from build123d import *

# Parameters (mm, degrees)
F0_R      = 18.4
F1_DEPTH  = 24
F2_R      = 17.25
F3_DEPTH  = 30
F4_R      = 6
F5_DEPTH  = 6.5
F6_R      = 3
F7_DEPTH  = 15.5
F8_SIZE   = 1
F10_DEPTH = 12
F12_D     = 3
F12_DEPTH = 24
F12_TIP   = 0.9012909285
F14_DEPTH = 1
F15_R     = 6.5
F16_DEPTH = 1.5
F17_SIZE  = 1
F18_W     = 3.175
F18_H     = 0.79375
F19_DEPTH = 5.6
F20_SIZE  = 1
F22_DEPTH = 25.4
F23_R     = 0.5


with BuildPart() as f1:
    # F0 (on Front) → F1 (new body)
    with BuildSketch(Plane.XZ):
        Circle(F0_R)
    extrude(amount=F1_DEPTH)

    # F2 (on face) → F3 (join)
    with BuildSketch(Plane(origin=(0, 0, 0), x_dir=(-1, 0, 0), z_dir=(0, 1, 0))):
        Circle(F2_R)
    extrude(amount=F3_DEPTH)

    # F4 (on face) → F5 (join)
    with BuildSketch(Plane.XZ.offset(24)):
        with Locations((7, 0)):
            Circle(F4_R)
    extrude(amount=F5_DEPTH)

    # F6 (on face) → F7 (join)
    with BuildSketch(Plane.XZ.offset(30.5)):
        with Locations((7, 0)):
            Circle(F6_R)
    extrude(amount=F7_DEPTH)

    # F8
    f8_edges = [f1.edges().sort_by_distance(p)[0] for p in [
        (1, -30.5, 0),
    ]]
    chamfer(f8_edges, length=F8_SIZE)

    # F9 (on face) → F10 (cut)
    with BuildSketch(Plane.XZ.offset(46)):
        with BuildLine():
            ThreePointArc((8.8, 2.4), (7, 3), (5.2, 2.4))
            Line((5.2, 2.4), (8.8, 2.4))
        make_face()
    extrude(amount=-F10_DEPTH, mode=Mode.SUBTRACT)

    # F12
    with Locations(Plane.XZ.offset(24)):
        with Locations((0, 15.5), (-13.4233937587, 7.75), (-13.4233937587, -7.75), (0, -15.5), (13.4233937587, -7.75), (13.4233937587, 7.75)):
            Hole(F12_D / 2, depth=F12_DEPTH)
            with Locations((0, 0, -(F12_DEPTH + F12_TIP / 2))):  # 118° drill point
                Cone(0, F12_D / 2, F12_TIP, mode=Mode.SUBTRACT)

    # F13 (on face) → F14 (cut)
    with BuildSketch(Plane.XZ.offset(24)):
        with BuildLine():
            ThreePointArc((7.1428571429, 7.9987243881), (8.1017881451, 8.6603638261), (7.7833850932, 9.7810488441))
            ThreePointArc((7.7833850932, 9.7810488441), (-12.5, 0), (7.7833850932, -9.7810488441))
            ThreePointArc((7.7833850932, -9.7810488441), (8.1017881451, -8.6603638261), (7.1428571429, -7.9987243881))
            ThreePointArc((7.1428571429, -7.9987243881), (-1, 0), (7.1428571429, 7.9987243881))
        make_face()
    extrude(amount=-F14_DEPTH, mode=Mode.SUBTRACT)

    # F15 (on face) → F16 (join)
    with BuildSketch(Plane(origin=(0, 30, 0), x_dir=(-1, 0, 0), z_dir=(0, 1, 0))):
        Circle(F15_R)
    extrude(amount=F16_DEPTH)

    # F17
    f17_edges = [f1.edges().sort_by_distance(p)[0] for p in [
        (6.5, 31.5, 0),
    ]]
    chamfer(f17_edges, length=F17_SIZE)

    # F18 (on face) → F19 (join)
    with BuildSketch(Plane(origin=(0, 30, 0), x_dir=(-1, 0, 0), z_dir=(0, 1, 0))):
        with Locations((0, 11.653125)):
            Rectangle(F18_W, F18_H)
        with Locations((0, -11.653125)):
            Rectangle(F18_W, F18_H)
    extrude(amount=F19_DEPTH)

    # F20
    f20_edges = [f1.edges().sort_by_distance(p)[0] for p in [
        (-1.5875, 35.6, 11.653125),
        (1.5875, 35.6, 11.653125),
        (1.5875, 35.6, -11.653125),
        (-1.5875, 35.6, -11.653125),
    ]]
    chamfer(f20_edges, length=F20_SIZE)

    # F21 (on face) → F22 (cut)
    with BuildSketch(Plane.XY.offset(12.05)):
        with BuildLine():
            Line((0.5, 33.04), (0.5, 34.31))
            ThreePointArc((0.5, 34.31), (0, 34.81), (-0.5, 34.31))
            Line((-0.5, 34.31), (-0.5, 33.04))
            ThreePointArc((-0.5, 33.04), (0, 32.54), (0.5, 33.04))
        make_face()
    extrude(amount=-F22_DEPTH, mode=Mode.SUBTRACT)

    # F23
    f23_edges = [f1.edges().sort_by_distance(p)[0] for p in [
        (-18.4, -24, 0),
    ]]
    fillet(f23_edges, radius=F23_R)


solid = f1.part
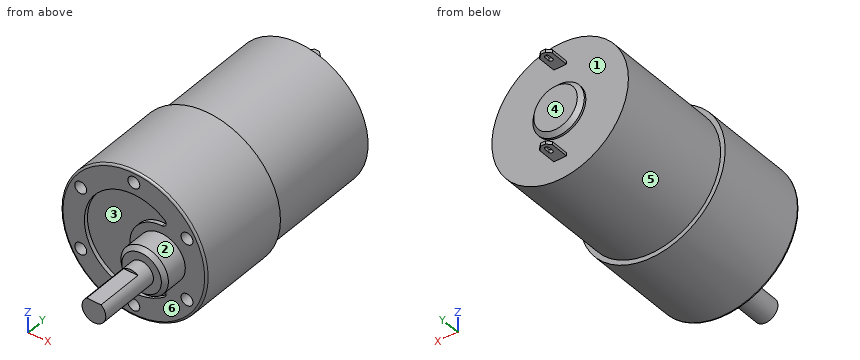
Input: part model. Units: mm. Frame: model coordinates. Face numbers are marked on the shaded views. A direction names the side the tool comes from. Round coordinates to 2 decimals unless told otherwise and drop trailing zeros. Order: outer loops, then holes, each group sorted by start corner. A loop starts at its lowest first (then second) coordinate and runs counter-clockwise, first axis right, second up. Notation, with made-up numbers: (76.25, 5.25) - (125.25, 5.25) arc R5 cw to (125.25, 13.25) - close; hole circle Ø2 at (49, 33.5). An arc over 180 degrees is marked (long way). Answer as a JSON object with one key per item and string values. Group by question number.
(1) Draft query along X for the marked faces 1, 2 and 3. Return one class per face: released by +X, released by -X, zero draft, split by the parting line, or undercut.
(2) Material intervals for probe 1 along Z at (x, y) = (0, -15.75); probe 2 along Y at (x, z) = (-3.5, 15.5); probe 3 along Z at (x, y) = (-13, -21.5), sorted ascending. Write a range as from..to.
(3) Reachability of the marked faces 4, 5 and 6 from +Z, -Z, +X, -X, +Y, -Y: full face, straight path, thin tool, end or side. Return the list, or none.
(4) Cut plane B-B (y = 25.5). Return loops of the section in (x, z), then the cut area to 3 significant figures.
(5) Pin query (flat end, axial travel): P1, Ø5, axis at x = 13.42, z = -7.75, coming from the +Y side; P2, Ø1, axis at x = -13.5, y = 7.5, coming from the +Z side; P3, Ø1.6, axis at x = 0, y = 34, coming from the -Z side. Return the tip coordinate at first contact, or that it passes through.
(6) Cut plane A-A (y = -38). Return loops of the section in (x, z), then the cut area to 3 significant figures.
Here are the results:
{
 "1": {"face 1": "zero draft", "face 2": "split by the parting line", "face 3": "undercut"},
 "2": {"probe 1": "z = -18.4..-17, -14..14, 17..18.4", "probe 2": "y = -24..30", "probe 3": "z = -13.02..-9.19, -6.31..6.31, 9.19..13.02"},
 "3": {"face 4": "+X, -X, +Y", "face 5": "+Y", "face 6": "-Y"},
 "4": {"outline": "circle Ø34.5 at (0, 0)", "area": "935 mm^2"},
 "5": {"P1": "stops at y = 30", "P2": "stops at z = 11.34", "P3": "stops at z = -12.05"},
 "6": {"outline": "(5.2, 2.4) arc R3 ccw (long way) to (8.8, 2.4) - close", "area": "26.8 mm^2"}
}
